Autodesk Inventor part; units mm, degrees
ref_plane "rod_cp_XY" through (0, 0, 0) normal (1, 0, 0) x (0, 0, -1)
ref_plane "rod_cp_YZ" through (0, 0, 0) normal (0, 0, -1) x (0, 1, 0)
ref_plane "rod_cp_ZX" through (0, 0, 0) normal (0, 1, 0) x (1, 0, 0)
sketch "Sketch_1" plane through (0, 0, 0) normal (0, 0, 1) x (1, 0, 0)
  line L0 (444.3984, 0) -> (-3.175, 0)
  line L1 (-3.175, 0) -> (-3.175, 3.9624)
  line L2 (-3.175, 3.9624) -> (422.275, 3.9624)
  line L3 (422.275, 3.9624) -> (422.275, 13.5572)
  line L4 (422.275, 13.5572) -> (444.3984, 13.5572)
  line L5 (444.3984, 13.5572) -> (444.3984, 0)
  line L6 (444.3984, 0) -> (-3.175, 0)
revolve "Revolution1" add sketch "Sketch_1" angle 360 about axis through (444.3984, 0, 0) along (1, 0, 0)
sketch "Sketch_3" plane through (0, 0, 0) normal (0, 0, 1) x (1, 0, 0)
  line L0 (-3.175, 0) -> (-15.875, 0)
  line L1 (-15.875, 0) -> (-15.875, 3.3388)
  line L2 (-15.875, 3.3388) -> (-15.2451, 3.9688)
  line L3 (-15.2451, 3.9688) -> (-3.175, 3.9688)
  line L4 (-3.175, 3.9688) -> (-3.175, 0)
  line L5 (-3.175, 0) -> (-15.875, 0)
revolve "Revolution2" add sketch "Sketch_3" angle 360 about axis through (-3.175, 0, 0) along (1, 0, 0)
thread "Thread1"
sketch "Sketch_10" plane through (-3.175, 0, 0) normal (1, 0, 0) x (0, 0, -1)
  line L0 (-7.9248, 7.9248) -> (-7.9248, -7.9248)
  line L1 (-7.9248, -7.9248) -> (7.9248, -7.9248)
  line L2 (7.9248, -7.9248) -> (7.9248, 7.9248)
  line L3 (7.9248, 7.9248) -> (-7.9248, 7.9248)
  line L4 (-3.175, 3.9624) -> (-3.175, -3.9624)
  line L5 (-3.175, -3.9624) -> (3.175, -3.9624)
  line L6 (3.175, -3.9624) -> (3.175, 3.9624)
  line L7 (3.175, 3.9624) -> (-3.175, 3.9624)
extrude "Extrusion1" cut sketch "Sketch_10" along normal blind 3.175
ref_plane "rod_cp_XY" through (0, 0, 0) normal (1, 0, 0) x (0, 0, -1)
ref_plane "rod_cp_YZ" through (0, 0, 0) normal (0, 0, -1) x (0, 1, 0)
ref_plane "rod_cp_ZX" through (0, 0, 0) normal (0, 1, 0) x (1, 0, 0)
ref_plane "to_rod_clevis_XY" through (-15.875, 0, 0) normal (1, 0, 0) x (0, 0, -1)
ref_plane "to_rod_clevis_YZ" through (-15.875, 0, 0) normal (0, 0, -1) x (0, 1, 0)
ref_plane "to_rod_clevis_ZX" through (-15.875, 0, 0) normal (0, 1, 0) x (1, 0, 0)
ref_plane "rl2_XY" through (-3.175, 0, 0) normal (1, 0, 0) x (0, 0, -1)
ref_plane "rl2_YZ" through (-3.175, 0, 0) normal (0, 0, -1) x (0, 1, 0)
ref_plane "rl2_ZX" through (-3.175, 0, 0) normal (0, 1, 0) x (1, 0, 0)
ref_plane "rl1_XY" through (-15.875, 0, 0) normal (1, 0, 0) x (0, 0, -1)
ref_plane "rl1_YZ" through (-15.875, 0, 0) normal (0, 0, -1) x (0, 1, 0)
ref_plane "rl1_ZX" through (-15.875, 0, 0) normal (0, 1, 0) x (1, 0, 0)
ref_plane "thd1_XY" through (-15.875, 3.9688, 0) normal (1, 0, 0) x (0, 0, -1)
ref_plane "thd1_YZ" through (-15.875, 3.9688, 0) normal (0, 0, -1) x (0, 1, 0)
ref_plane "thd1_ZX" through (-15.875, 3.9688, 0) normal (0, 1, 0) x (1, 0, 0)
ref_plane "thd2_XY" through (-15.875, -3.9688, 0) normal (1, 0, 0) x (0, 0, -1)
ref_plane "thd2_YZ" through (-15.875, -3.9688, 0) normal (0, 0, -1) x (0, 1, 0)
ref_plane "thd2_ZX" through (-15.875, -3.9688, 0) normal (0, 1, 0) x (1, 0, 0)
ref_plane "dia1_XY" through (-3.175, 3.9624, 0) normal (1, 0, 0) x (0, 0, -1)
ref_plane "dia1_YZ" through (-3.175, 3.9624, 0) normal (0, 0, -1) x (0, 1, 0)
ref_plane "dia1_ZX" through (-3.175, 3.9624, 0) normal (0, 1, 0) x (1, 0, 0)
ref_plane "dia2_XY" through (-3.175, -3.9624, 0) normal (1, 0, 0) x (0, 0, -1)
ref_plane "dia2_YZ" through (-3.175, -3.9624, 0) normal (0, 0, -1) x (0, 1, 0)
ref_plane "dia2_ZX" through (-3.175, -3.9624, 0) normal (0, 1, 0) x (1, 0, 0)
ref_plane "wf1_XY" through (-3.175, 0, 0) normal (1, 0, 0) x (0, 0, -1)
ref_plane "wf1_YZ" through (-3.175, 0, 0) normal (0, 0, -1) x (0, 1, 0)
ref_plane "wf1_ZX" through (-3.175, 0, 0) normal (0, 1, 0) x (1, 0, 0)
ref_plane "wf2_XY" through (0, 0, 0) normal (1, 0, 0) x (0, 0, -1)
ref_plane "wf2_YZ" through (0, 0, 0) normal (0, 0, -1) x (0, 1, 0)
ref_plane "wf2_ZX" through (0, 0, 0) normal (0, 1, 0) x (1, 0, 0)
ref_plane "hh1_XY" through (472.1606, 0, 0) normal (0, 0, 1) x (1, 0, 0)
ref_plane "hh1_YZ" through (472.1606, 0, 0) normal (1, 0, 0) x (0, 1, 0)
ref_plane "hh1_ZX" through (472.1606, 0, 0) normal (0, 1, 0) x (0, 0, 1)
ref_plane "hh2_XY" through (478.5614, 0, 0) normal (0, 0, 1) x (1, 0, 0)
ref_plane "hh2_YZ" through (478.5614, 0, 0) normal (1, 0, 0) x (0, 1, 0)
ref_plane "hh2_ZX" through (478.5614, 0, 0) normal (0, 1, 0) x (0, 0, 1)
ref_plane "dia12_XY" through (0, 0, 14.1351) normal (1, 0, 0) x (0, 0, -1)
ref_plane "dia12_YZ" through (0, 0, 14.1351) normal (0, 0, -1) x (0, 1, 0)
ref_plane "dia12_ZX" through (0, 0, 14.1351) normal (0, 1, 0) x (1, 0, 0)
ref_plane "dia22_XY" through (0, 0, -14.1351) normal (1, 0, 0) x (0, 0, -1)
ref_plane "dia22_YZ" through (0, 0, -14.1351) normal (0, 0, -1) x (0, 1, 0)
ref_plane "dia22_ZX" through (0, 0, -14.1351) normal (0, 1, 0) x (1, 0, 0)
ref_plane "wfw1_XY" through (-3.175, 0, -3.175) normal (0, 1, 0) x (1, 0, 0)
ref_plane "wfw1_YZ" through (-3.175, 0, -3.175) normal (1, 0, 0) x (0, 0, -1)
ref_plane "wfw1_ZX" through (-3.175, 0, -3.175) normal (0, 0, -1) x (0, 1, 0)
ref_plane "wfw2_XY" through (-3.175, 0, 3.175) normal (0, 1, 0) x (1, 0, 0)
ref_plane "wfw2_YZ" through (-3.175, 0, 3.175) normal (1, 0, 0) x (0, 0, -1)
ref_plane "wfw2_ZX" through (-3.175, 0, 3.175) normal (0, 0, -1) x (0, 1, 0)
properties part number "0915-DX0_rod"
The model under review builds one solid part; all positions refer to its coordinate system, in mm. A direction names the side the tool comes from. Coordinates: 2 decimals unless noted, no trailing zeros. Write each loop counter-clockwise with the first axis right and the second up, starting at its lowest first coordinate (ties: lowest second). Pieces come first, ordered by that corner, then holes. Notation, with made-up numbers: (-39.75, 70) - (6.25, 70) arc R6 ccw to (6.25, 77) - close; hole circle Ø10 at (-22, -27). An arc over 180 degrees is marked (long way). Write item = value, one per line.
(1) Consider section B-B, the plane z = -9.25. Give the boundary of the cut face in (x, y) (3 decimals).
Result sheet:
outline = (422.275, -9.911) - (444.398, -9.911) - (444.398, 9.911) - (422.275, 9.911) - close
(2) Machinability: for faces 1 (the face through (-9.126, 3.666, -1.52)), 2 (the face through (444.398, 0, 0)), which of the approach directions +Z, -Z, +X, -X, +Y, -Y give a long, thin tool a straight path to every point of the face, cutting with its end or side? Answer none if there is none.
Result sheet:
face_1 = -X
face_2 = +Z, -Z, +X, +Y, -Y
(3) For line 1 (X direction, y = 6.5, z = 5.25) (3 decimals); line 2 (Y direction, x = 220, z = 2.25); line 3 (Z direction, x = 22, y = 1.75), list the stretches that pass through material, from the lowest coordinate up. Write a range as [from, to].
Result sheet:
line_1 = [422.275, 444.398]
line_2 = [-3.26, 3.26]
line_3 = [-3.56, 3.56]
(4) For P1, Ø5, axis at x = 299.5, y = 7, coming from the -Z side; P2, Ø3, axis at y = 7, z = -9, coming from the -X side (3 decimals); P3, Ø3.5, axis at x = -2, y = 1, coming from the +Z side; P4, Ø1.6, axis at x = -2, y = 0.5, coming from the -Z side (3 decimals), all flat-tipped, find the tip position at first contact; note any pin that passes through.
Result sheet:
P1 = through
P2 = 422.275
P3 = 3.97
P4 = -3.175
(5) Consider section A-A, the plane x = 28.5. Give the boundary of the cut face in (y, z), then the cut area to 3 significant figures.
Result sheet:
outline = circle Ø7.92 at (0, 0)
area = 49.3 mm^2
